```python
from build123d import *

# Parameters (mm, degrees)
SKETCH1_R           = 2.5
BOSS_EXTRUDE3_DEPTH = 8
BOSS_EXTRUDE7_DEPTH = 5
CUT_EXTRUDE1_DEPTH  = 112.404667766
SKETCH18_R          = 1.55
CUT_EXTRUDE2_DEPTH  = 6
CUT_EXTRUDE3_START  = -6
SKETCH19_R          = 1.55
CUT_EXTRUDE3_DEPTH  = 6
SKETCH21_R          = 22
CUT_EXTRUDE5_DEPTH  = 5


with BuildPart() as part:
    # Sketch1 → Boss-Extrude3 (new body)
    # profile 1 of 5: a face of its own
    with BuildSketch(Plane.XY):
        with BuildLine():
            Line((-66.254964627, 19), (-90, -19))
            Line((-90, -19), (90, -19))
            ThreePointArc((90, -19), (71, 0), (90, 19))
            Line((90, 19), (-66.254964627, 19))
        make_face()
        with Locations((-50, 0)):
            Circle(SKETCH1_R, mode=Mode.SUBTRACT)
        with BuildLine():
            ThreePointArc((40, -7.5), (39.267766953, -9.267766953), (37.5, -10))
            Line((37.5, -10), (2.5, -10))
            ThreePointArc((2.5, -10), (0.732233047, -9.267766953), (0, -7.5))
            Line((0, -7.5), (0, 7.5))
            ThreePointArc((0, 7.5), (0.732233047, 9.267766953), (2.5, 10))
            Line((2.5, 10), (37.5, 10))
            ThreePointArc((37.5, 10), (39.267766953, 9.267766953), (40, 7.5))
            Line((40, 7.5), (40, -7.5))
        make_face(mode=Mode.SUBTRACT)
    # profile 2 of 5: a face of its own
    with BuildSketch(Plane.XY):
        with BuildLine():
            ThreePointArc((90, 19), (71, 0), (90, -19))
            Line((90, -19), (90, -2.5))
            ThreePointArc((90, -2.5), (87.5, 0), (90, 2.5))
            Line((90, 2.5), (90, 19))
        make_face()
    # profile 3 of 5: a face of its own
    with BuildSketch(Plane.XY):
        with BuildLine():
            Line((90, -2.5), (90, -19))
            ThreePointArc((90, -19), (103.435028843, -13.435028843), (109, 0))
            ThreePointArc((109, 0), (103.435028843, 13.435028843), (90, 19))
            Line((90, 19), (90, 2.5))
            ThreePointArc((90, 2.5), (91.767766953, 1.767766953), (92.5, 0))
            ThreePointArc((92.5, 0), (91.767766953, -1.767766953), (90, -2.5))
        make_face()
    # profile 4 of 5: a face of its own
    with BuildSketch(Plane.XY):
        with BuildLine():
            ThreePointArc((90, 19), (71, 0), (90, -19))
            Line((90, -19), (90, -2.5))
            ThreePointArc((90, -2.5), (87.5, 0), (90, 2.5))
            Line((90, 2.5), (90, 19))
        make_face()
    # profile 5 of 5: a face of its own
    with BuildSketch(Plane.XY):
        with BuildLine():
            Line((90, -2.5), (90, -19))
            ThreePointArc((90, -19), (103.435028843, -13.435028843), (109, 0))
            ThreePointArc((109, 0), (103.435028843, 13.435028843), (90, 19))
            Line((90, 19), (90, 2.5))
            ThreePointArc((90, 2.5), (91.767766953, 1.767766953), (92.5, 0))
            ThreePointArc((92.5, 0), (91.767766953, -1.767766953), (90, -2.5))
        make_face()
    extrude(amount=BOSS_EXTRUDE3_DEPTH)

    # Sketch3 → Boss-Extrude7 (add)
    with BuildSketch(Plane.XY.offset(8)):
        with BuildLine():
            Line((-32.948367789, 19), (72.948367789, 19))
            ThreePointArc((72.948367789, 19), (74.716134742, 18.267766953), (75.448367789, 16.5))
            Line((75.448367789, 16.5), (75.448367789, -16.5))
            ThreePointArc((75.448367789, -16.5), (74.716134742, -18.267766953), (72.948367789, -19))
            Line((72.948367789, -19), (-32.948367789, -19))
            ThreePointArc((-32.948367789, -19), (-34.716134742, -18.267766953), (-35.448367789, -16.5))
            Line((-35.448367789, -16.5), (-35.448367789, 16.5))
            ThreePointArc((-35.448367789, 16.5), (-34.716134742, 18.267766953), (-32.948367789, 19))
        make_face()
    extrude(amount=BOSS_EXTRUDE7_DEPTH)

    # Sketch14 → Cut-Extrude1 (cut, through all)
    with BuildSketch(Plane.XY.offset(13)):
        with BuildLine():
            Line((2.5, -10), (37.5, -10))
            ThreePointArc((37.5, -10), (39.267766953, -9.267766953), (40, -7.5))
            Line((40, -7.5), (40, 7.5))
            ThreePointArc((40, 7.5), (39.267766953, 9.267766953), (37.5, 10))
            Line((37.5, 10), (2.5, 10))
            ThreePointArc((2.5, 10), (0.732233047, 9.267766953), (0, 7.5))
            Line((0, 7.5), (0, -7.5))
            ThreePointArc((0, -7.5), (0.732233047, -9.267766953), (2.5, -10))
        make_face()
    extrude(amount=-CUT_EXTRUDE1_DEPTH, mode=Mode.SUBTRACT)

    # Sketch18 → Cut-Extrude2 (cut)
    with BuildSketch(Plane.XZ.offset(19)):
        with Locations((-23.89, 6.5)):
            Circle(SKETCH18_R)
        with Locations((20, 6.5)):
            Circle(SKETCH18_R)
        with Locations((63.89, 6.5)):
            Circle(SKETCH18_R)
    extrude(amount=-CUT_EXTRUDE2_DEPTH, mode=Mode.SUBTRACT)

    # Sketch19 → Cut-Extrude3 (cut)
    with BuildSketch(Plane(origin=(0, 19, 0), x_dir=(1, 0, 0), z_dir=(0, 1, 0)).offset(CUT_EXTRUDE3_START)):
        with Locations((-23.89, -6.5)):
            Circle(SKETCH19_R)
        with Locations((20, -6.5)):
            Circle(SKETCH19_R)
        with Locations((63.89, -6.5)):
            Circle(SKETCH19_R)
    extrude(amount=CUT_EXTRUDE3_DEPTH, mode=Mode.SUBTRACT)

    # Sketch21 → Cut-Extrude5 (cut)
    with BuildSketch(Plane.XY.offset(13)):
        with Locations((-50, 0)):
            Circle(SKETCH21_R)
        with Locations((90, 0)):
            Circle(SKETCH21_R)
    extrude(amount=-CUT_EXTRUDE5_DEPTH, mode=Mode.SUBTRACT)


solid = part.part
```
CAD build for the part. Positions are in the model's coordinates, mm. A direction names the side the tool comes from. Coordinates: 2 decimals unless noted, no trailing zeros. Write each loop counter-clockwise with the first axis right and the second up, starting at its lowest first coordinate (ties: lowest second). Pieces come first, ordered by that corner, then holes.
(1) Drill centre lines: probe 1 along Y at (x, z) = (7.5, 4.25); probe 2 along Z at (x, y) = (63.89, -16.05); probe 3 along X at (y, z) = (1, 0.5). Where is each one in solid material? Low to high.
(2) 3-axis set-ups, long thin cutter, end or side, ignore diameter. For faces 1 (the face through (21.432, -16.042, 5.906)), 2 (the face through (21.432, 15.958, 7.094)), 3 (the face through (20, -10, 7)): which of +Z, -Z, +X, -X, +Y, -Y reach the whole face in a straight line?
(3) Cut at B-B, the plane z = 2.5. List the corners of the cut face in (x, y), and give its area (3 significant figures).
(4) Two-plate mould, pull along Z, no slides. Class faces 4 (the face through (64, 13, 6)), 5 (the face through (20, 10, 7)): +Z half, -Z half, draft (parallel to the pull), parting line (faces both ways), or undercut.
(5) Flat gauge pins, fed straight in: pin 1 (6 mm diameter, centred on x = -42.5, y = 13, fed in from +Z); pin 2 (1.9 mm diameter, centred on x = -23.89, z = 6.5, fed in from -Y); pin 3 (0.9 mm diameter, centred on x = 63.5, z = 7, fed in from +Y). Where does each tip first touch, or does it go through?
(6) Cut at A-A, the plane x = -50. List the corners of the cut face in (y, z), and give its area (3 significant figures).
(7) Cut at C-C, the plane z = 11. List the corners of the cut face in (x, y), and give its area (3 significant figures).
Geometry says:
1. probe 1: y = -19 to -10, 10 to 19
1. probe 2: z = 0 to 4.95, 8.05 to 13
1. probe 3: x = -77.5 to -52.29, -47.71 to 0, 40 to 87.71, 92.29 to 108.97
2. face 1: -Y
2. face 2: +Y
2. face 3: +Z, -Z
3. outline: (-90, -19) - (90, -19) arc R19 ccw to (90, 19) - (-66.25, 19) - close; hole circle Ø5 at (-50, 0); hole (0, -7.5) arc R2.5 ccw to (2.5, -10) - (37.5, -10) arc R2.5 ccw to (40, -7.5) - (40, 7.5) arc R2.5 ccw to (37.5, 10) - (2.5, 10) arc R2.5 ccw to (0, 7.5) - close; hole circle Ø5 at (90, 0)
3. area: 6,120 mm2
4. face 4: undercut
4. face 5: draft
5. pin 1: stops at z = 8
5. pin 2: stops at y = -13
5. pin 3: stops at y = 13
6. outline: (-19, 0) - (-2.5, 0) - (-2.5, 8) - (-19, 8) - close; (2.5, 0) - (19, 0) - (19, 8) - (2.5, 8) - close
6. area: 264 mm2
7. outline: (-35.45, -16.5) arc R2.5 ccw to (-32.95, -19) - (72.95, -19) arc R2.5 ccw to (75.45, -16.5) arc R22 cw to (75.45, 16.5) arc R2.5 ccw to (72.95, 19) - (-32.95, 19) arc R2.5 ccw to (-35.45, 16.5) arc R22 cw to start; hole (0, -7.5) arc R2.5 ccw to (2.5, -10) - (37.5, -10) arc R2.5 ccw to (40, -7.5) - (40, 7.5) arc R2.5 ccw to (37.5, 10) - (2.5, 10) arc R2.5 ccw to (0, 7.5) - close
7. area: 3,070 mm2
